The listing builds one solid part. Answer for the finished solid, in the listing's coordinates (mm). A direction names the side the tool comes from. Coordinates: 2 decimals unless noted, no trailing zeros. Order: outer loops, then holes, each group sorted by start corner. A loop starts at its lowest first (then second) coordinate and runs counter-clockwise, first axis right, second up. Notation, with made-up numbers: (37, 56.5) -> (56, 56.5) arc R21 cw to (56, 73.5) -> close; hole circle Ø7 at (88, -33.5). An arc over 180 degrees is marked (long way). Answer in a Markdown table with one row per item.
```python
from build123d import *

# Parameters (mm, degrees)
SKETCH034_W          = 59.2
SKETCH034_H          = 53.7
SKETCH034_R          = 1.75
PAD011_DEPTH         = 1.6
SKETCH032_W          = 55.7
SKETCH032_H          = 53.7
SKETCH032_W_2        = 52.5
SKETCH032_H_2        = 50.5
PAD010_DEPTH         = 40
CHAMFER001_SIZE      = 1.15
FILLET004_R          = 1
SKETCH033_W          = 5
SKETCH033_H          = 3
SKETCH033_W_2        = 5.25
SKETCH033_H_2        = 2.5
POCKET007_DEPTH      = 31.351
POCKET007_DEPTH_BACK = 27.851
POCKET_DEPTH         = 31.351
POCKET041_DEPTH      = 27.851
SKETCH030_W          = 9
SKETCH030_H          = 4
POCKET009_DEPTH      = 26.851
POCKET009_DEPTH_BACK = 26.851
SKETCH029_R          = 3.2
PAD009_DEPTH         = 2.2
SKETCH050_R          = 1.75
POCKET015_DEPTH      = 3.801
SKETCH036_W          = 0.4
SKETCH036_H          = 1.5
POCKET008_DEPTH      = 8


with BuildPart() as part:
    # Sketch034 → Pad011 (new body)
    with BuildSketch(Plane.XY):
        with Locations((-1.75, 0)):
            Rectangle(SKETCH034_W, SKETCH034_H)
        with Locations((19.652, 0)):
            Circle(SKETCH034_R, mode=Mode.SUBTRACT)
    extrude(amount=PAD011_DEPTH)

    # Sketch032 → Pad010 (join)
    with BuildSketch(Plane.XY.offset(1.6)):
        Rectangle(SKETCH032_W, SKETCH032_H)
        Rectangle(SKETCH032_W_2, SKETCH032_H_2, mode=Mode.SUBTRACT)
    extrude(amount=PAD010_DEPTH)

    # Chamfer001
    chamfer001_edges = [part.edges().sort_by_distance(p)[0] for p in [
        (26.25, 0, 41.6),
        (-26.25, 0, 41.6),
    ]]
    chamfer(chamfer001_edges, length=CHAMFER001_SIZE)

    # Fillet004
    fillet004_edges = [part.edges().sort_by_distance(p)[0] for p in [
        (26.25, -25.25, 21.025),
        (-26.25, -25.25, 21.025),
        (27.85, -26.85, 21.6),
        (-26.25, 25.25, 21.025),
        (-27.85, -26.85, 21.6),
        (26.25, 25.25, 21.025),
        (0, -25.25, 1.6),
        (0, 25.25, 1.6),
        (-27.85, 26.85, 21.6),
        (27.85, 26.85, 21.6),
        (-26.25, 0, 1.6),
        (26.25, 0, 1.6),
        (-31.35, -26.85, 0.8),
        (-31.35, 26.85, 0.8),
    ]]
    fillet(fillet004_edges, radius=FILLET004_R)

    # Sketch033 → Pocket007 (cut, two sides)
    with BuildSketch(Plane.YZ) as pocket007_sk:
        with Locations((-15, 36.1)):
            Rectangle(SKETCH033_W, SKETCH033_H)
        with Locations((15, 36.1)):
            Rectangle(SKETCH033_W, SKETCH033_H)
        with Locations((-9.125, 40.35)):
            Rectangle(SKETCH033_W_2, SKETCH033_H_2)
        with Locations((9.125, 40.35)):
            Rectangle(SKETCH033_W_2, SKETCH033_H_2)
    extrude(amount=-POCKET007_DEPTH, mode=Mode.SUBTRACT)
    extrude(pocket007_sk.sketch, amount=POCKET007_DEPTH_BACK, mode=Mode.SUBTRACT)

    # Sketch109 → Pocket (cut, through all)
    with BuildSketch(Plane.YZ):
        with BuildLine():
            Line((-23.733, 17.8), (-23.733, 1.6))
            Line((-23.733, 1.6), (23.733, 1.6))
            Line((23.733, 1.6), (23.733, 17.8))
            ThreePointArc((23.733, 17.8), (22.268534, 21.335534), (18.733, 22.8))
            Line((-18.733, 22.8), (18.733, 22.8))
            ThreePointArc((-18.733, 22.8), (-22.268534, 21.335534), (-23.733, 17.8))
        make_face()
    extrude(amount=-POCKET_DEPTH, mode=Mode.SUBTRACT)

    # Sketch110 → Pocket041 (cut, through all)
    with BuildSketch(Plane.YZ):
        with BuildLine():
            Line((-22.733, 18.6), (-15.733, 18.6))
            ThreePointArc((-14.733, 17.6), (-15.025893, 18.307107), (-15.733, 18.6))
            Line((-14.733, 17.6), (-14.733, 10.6))
            ThreePointArc((-15.733, 9.6), (-15.025893, 9.892893), (-14.733, 10.6))
            Line((-15.733, 9.6), (-22.733, 9.6))
            ThreePointArc((-23.733, 10.6), (-23.440107, 9.892893), (-22.733, 9.6))
            Line((-23.733, 10.6), (-23.733, 17.6))
            ThreePointArc((-22.733, 18.6), (-23.440107, 18.307107), (-23.733, 17.6))
        make_face()
        with BuildLine():
            Line((22.733, 18.6), (15.733, 18.6))
            ThreePointArc((15.733, 18.6), (15.025893, 18.307107), (14.733, 17.6))
            Line((14.733, 17.6), (14.733, 10.6))
            ThreePointArc((14.733, 10.6), (15.025893, 9.892893), (15.733, 9.6))
            Line((15.733, 9.6), (22.733, 9.6))
            ThreePointArc((22.733, 9.6), (23.440107, 9.892893), (23.733, 10.6))
            Line((23.733, 10.6), (23.733, 17.6))
            ThreePointArc((23.733, 17.6), (23.440107, 18.307107), (22.733, 18.6))
        make_face()
    extrude(amount=POCKET041_DEPTH, mode=Mode.SUBTRACT)

    # Sketch030 → Pocket009 (cut, two sides)
    with BuildSketch(Plane.XZ) as pocket009_sk:
        with Locations((-16, 39.6)):
            Rectangle(SKETCH030_W, SKETCH030_H)
        with Locations((16, 39.6)):
            Rectangle(SKETCH030_W, SKETCH030_H)
    extrude(amount=-POCKET009_DEPTH, mode=Mode.SUBTRACT)
    extrude(pocket009_sk.sketch, amount=POCKET009_DEPTH_BACK, mode=Mode.SUBTRACT)

    # Sketch029 → Pad009 (join)
    with BuildSketch(Plane.XY.offset(1.6)):
        with Locations((-28.048, 15.621)):
            Circle(SKETCH029_R)
        with Locations((-15.348, 15.621)):
            Circle(SKETCH029_R)
        with Locations((-15.348, -19.431)):
            Circle(SKETCH029_R)
        with Locations((-28.048, -19.431)):
            Circle(SKETCH029_R)
    extrude(amount=PAD009_DEPTH)

    # Sketch050 → Pocket015 (cut, through all)
    with BuildSketch(Plane.XY.offset(3.8)):
        with Locations((-28.048, 15.621)):
            Circle(SKETCH050_R)
        with Locations((-15.348, 15.621)):
            Circle(SKETCH050_R)
        with Locations((-15.348, -19.431)):
            Circle(SKETCH050_R)
        with Locations((-28.048, -19.431)):
            Circle(SKETCH050_R)
    extrude(amount=-POCKET015_DEPTH, mode=Mode.SUBTRACT)

    # Sketch036 → Pocket008 (cut)
    with BuildSketch(Plane.XY.offset(41.6)):
        with Locations((-26.45, 21.5)):
            Rectangle(SKETCH036_W, SKETCH036_H)
        with Locations((26.45, 21.5)):
            Rectangle(SKETCH036_W, SKETCH036_H)
        with Locations((-26.45, -21.5)):
            Rectangle(SKETCH036_W, SKETCH036_H)
        with Locations((26.45, -21.5)):
            Rectangle(SKETCH036_W, SKETCH036_H)
    extrude(amount=-POCKET008_DEPTH, mode=Mode.SUBTRACT)


solid = part.part
```
(1) Flat-ended cylindrical pins translate along their axes: pin 1 (12 mm diameter, centred on x = -13.5, y = 5.5, fed in from +Z); pin 2 (1 mm diameter, centred on y = -8, z = 11, fed in from -X); pin 3 (0.8 mm diameter, centred on y = -26, z = 40.5, fed in from -X); pin 4 (5 mm diameter, centred on x = -29.5, y = 14, fed in from +Z). Find the tip coordinate at first contact, or state that the pin passes through.
Check values:
| item | result |
|---|---|
| pin 1 | z = 1.6 |
| pin 2 | x = 26.25 |
| pin 3 | x = -27.85 |
| pin 4 | z = 41.6 |
(2) A cutting plane is placed at B-B, the plane y = -10.5. Determine the outline of the cut face in (x, z), then the cut area to 3 significant figures.
Check values:
| item | result |
|---|---|
| outline | (-31.35, 0) -> (27.85, 0) -> (27.85, 39.1) -> (26.25, 39.1) -> (26.25, 2.6) arc R1 cw to (25.25, 1.6) -> (-31.35, 1.6) -> close; (-27.85, 22.8) -> (-26.25, 22.8) -> (-26.25, 39.1) -> (-27.85, 39.1) -> close |
| area | 181 mm² |
(3) Find the intervals of material crossed by line 1 along X through (y, z) = (-2, 37.5); line 2 along Y through (x, z) = (-6.5, 28.5); line 3 along X through (y, z) = (-17.5, 3.5), in increasing order. Write a range as from..to.
Check values:
| item | result |
|---|---|
| line 1 | -27.85..-26.25, 26.25..27.85 |
| line 2 | -26.85..-25.25, 25.25..26.85 |
| line 3 | -30.6..-25.5, -17.9..-12.8, 26.25..27.85 |
(4) A cutting plane is placed at D-D, the plane y = 0. Determine the outline of the cut face in (x, z), then the cut area to 3 significant figures.
Check values:
| item | result |
|---|---|
| outline | (-31.35, 0) -> (17.9, 0) -> (17.9, 1.6) -> (-31.35, 1.6) -> close; (-27.85, 22.8) -> (-26.25, 22.8) -> (-26.25, 40.45) -> (-27.4, 41.6) -> (-27.85, 41.6) -> close; (21.4, 0) -> (27.85, 0) -> (27.85, 41.6) -> (27.4, 41.6) -> (26.25, 40.45) -> (26.25, 2.6) arc R1 cw to (25.25, 1.6) -> (21.4, 1.6) -> close |
| area | 182 mm² |
(5) A cutting plane is placed at A-A, the plane z = 15.5. Determine the outline of the cut face in (x, y), then the cut area to 3 significant figures.
Check values:
| item | result |
|---|---|
| outline | (-27.85, -25.85) arc R1 ccw to (-26.85, -26.85) -> (26.85, -26.85) arc R1 ccw to (27.85, -25.85) -> (27.85, -23.73) -> (26.25, -23.73) -> (26.25, -24.25) arc R1 cw to (25.25, -25.25) -> (-25.25, -25.25) arc R1 cw to (-26.25, -24.25) -> (-26.25, -23.73) -> (-27.85, -23.73) -> close; (-27.85, 23.73) -> (-26.25, 23.73) -> (-26.25, 24.25) arc R1 cw to (-25.25, 25.25) -> (25.25, 25.25) arc R1 cw to (26.25, 24.25) -> (26.25, 23.73) -> (27.85, 23.73) -> (27.85, 25.85) arc R1 ccw to (26.85, 26.85) -> (-26.85, 26.85) arc R1 ccw to (-27.85, 25.85) -> close; (26.25, -14.73) -> (27.85, -14.73) -> (27.85, 14.73) -> (26.25, 14.73) -> close |
| area | 235 mm² |
(6) A cutting plane is placed at C-C, the plane z = 31. Determine the outline of the cut face in (x, y), then the cut area to 3 significant figures.
Check values:
| item | result |
|---|---|
| outline | (-27.85, -25.85) arc R1 ccw to (-26.85, -26.85) -> (26.85, -26.85) arc R1 ccw to (27.85, -25.85) -> (27.85, 25.85) arc R1 ccw to (26.85, 26.85) -> (-26.85, 26.85) arc R1 ccw to (-27.85, 25.85) -> close; hole (-26.25, -24.25) arc R1 ccw to (-25.25, -25.25) -> (25.25, -25.25) arc R1 ccw to (26.25, -24.25) -> (26.25, 24.25) arc R1 ccw to (25.25, 25.25) -> (-25.25, 25.25) arc R1 ccw to (-26.25, 24.25) -> close |
| area | 340 mm² |
(7) For a pull along X with two mould halves and no side action, classify faces 5 (the cylindrical face through (-30.587, -21.378, 2.685)), 6 (the flat face through (27, 11.75, 40)), 7 (the flat face through (-31.35, 0, 1)) as released by +X, released by -X, zero draft, split by the parting line, or undercut.
Check values:
| item | result |
|---|---|
| face 5 | undercut |
| face 6 | zero draft |
| face 7 | released by -X |
(8) Which of the six approach directions +Z, -Z, +X, -X, +Y, -Y give full straight-line access (tool end or side, diameter ignored) to faces 1 (the flat face through (27, 15, 37.6)), 2 (the flat face through (-26.65, 21, 37)), 3 (the flat face through (11.5, -26, 40)), 4 (the flat face through (-27, -23.733, 10))?
Check values:
| item | result |
|---|---|
| face 1 | +X, -X |
| face 2 | +Z |
| face 3 | +Z, +Y, -Y |
| face 4 | -X |
